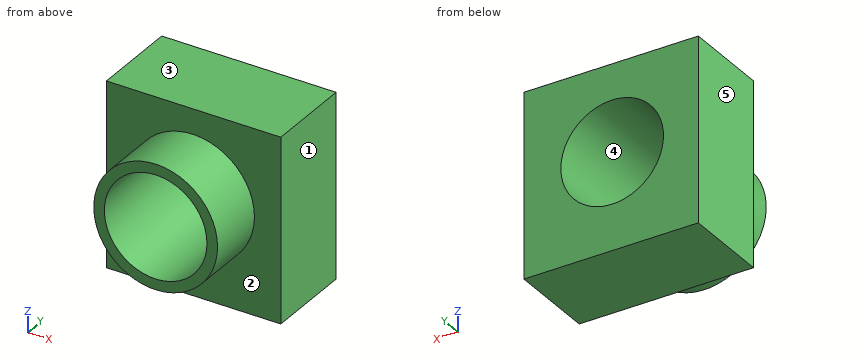
```python
from build123d import *

# Parameters (mm, degrees)
F0_W     = 75.738185
F0_H     = 79.894543
F1_DEPTH = 38.1
F2_R     = 26.877172
F3_DEPTH = 25.4
F4_R     = 22.28871
F5_DEPTH = 63.501


with BuildPart() as f1:
    # F0 (on Front) → F1 (new body)
    with BuildSketch(Plane.XZ):
        with Locations((0.46182, -2.193634)):
            Rectangle(F0_W, F0_H)
    extrude(amount=F1_DEPTH)

    # F2 (on face) → F3 (join)
    with BuildSketch(Plane.XZ.offset(38.1)):
        Circle(F2_R)
    extrude(amount=F3_DEPTH)

    # F4 (on face) → F5 (cut, through all)
    with BuildSketch(Plane.XZ.offset(63.5)):
        Circle(F4_R)
    extrude(amount=-F5_DEPTH, mode=Mode.SUBTRACT)


solid = f1.part
```
The listing builds one solid part. Answer for the finished solid, in the listing's coordinates (mm). Face numbers are marked on the shaded views. A direction names the side the tool comes from. Coordinates: 2 decimals unless noted, no trailing zeros. Loops run counter-clockwise (first coordinate to the right, second up) from the corner with the lowest first, then second, coordinate; pieces in that order, holes last. Notation, with made-up numbers: M 22,41 L 64,41 A8 ccw 64,53 Z; hole C 54,-12 d2. An arc over 180 degrees is marked long. Answer as a JSON object with one key per item and string values. Group by question number.
Item 1: Section C-C (y = -30.5) is taken. Write down the section's boundary in (x, z).
Item 2: Determine the mould class of the marked faces 3, 4 and 5 for opening direction X: +X half, -X half, draft (parallel to the pull), parting line (faces both ways), or undercut.
Item 3: Consider L1, parallel to Z at x = 0, y = -27.5; L2, parallel to Z at x = 0, y = -47.5; L3, parallel to X at y = -8.5, z = 16. Determine where each line is inside the solid, lowest interval first.
Item 4: Section B-B (x = 0) is taken. Write down the section's boundary in (y, z), and give its area (3 significant figures).
Item 5: Section D-D (x = 24) is taken. Write down the section's boundary in (y, z).
Item 6: Section A-A (z = 0) is taken. Write down the section's boundary in (x, y), and give its area (3 significant figures).
Item 7: Each of these flat-tipped pins is pushed along its axis until it touches: P1, Ø12, axis at x = 15, z = -32, coming from the -Y side; P2, Ø22.5, axis at x = -18.5, z = -20.5, coming from the -Y side; P3, Ø1.5, axis at y = -46.5, z = -22.5, coming from the +X side; P4, Ø1, axis at x = -14.5, z = -14, coming from the +Y side. Where does it stop, or does it pass through?
Item 8: Which of the six approach directions +Z, -Z, +X, -X, +Y, -Y give full straight-line access (tool end or side, diameter ignored) to the marked faces 1 and 2?
Solved:
{
 "1": {"outline": "M -37.41,-42.14 L 38.33,-42.14 L 38.33,37.75 L -37.41,37.75 Z; hole C 0,0 d44.58"},
 "2": {"face 3": "draft", "face 4": "undercut", "face 5": "-X half"},
 "3": {"L1": "z = -42.14 to -22.29, 22.29 to 37.75", "L2": "z = -26.88 to -22.29, 22.29 to 26.88", "L3": "x = -37.41 to -15.52, 15.52 to 38.33"},
 "4": {"outline": "M -63.5,-26.88 L -38.1,-26.88 L -38.1,-42.14 L 0,-42.14 L 0,-22.29 L -63.5,-22.29 Z; M -63.5,22.29 L 0,22.29 L 0,37.75 L -38.1,37.75 L -38.1,26.88 L -63.5,26.88 Z", "area": "1,580 mm2"},
 "5": {"outline": "M -63.5,-12.1 L -38.1,-12.1 L -38.1,-42.14 L 0,-42.14 L 0,37.75 L -38.1,37.75 L -38.1,12.1 L -63.5,12.1 Z"},
 "6": {"outline": "M -37.41,-38.1 L -26.88,-38.1 L -26.88,-63.5 L -22.29,-63.5 L -22.29,0 L -37.41,0 Z; M 22.29,-63.5 L 26.88,-63.5 L 26.88,-38.1 L 38.33,-38.1 L 38.33,0 L 22.29,0 Z", "area": "1,420 mm2"},
 "7": {"P1": "stops at y = -38.1", "P2": "stops at y = -63.5", "P3": "stops at x = 15.79", "P4": "passes through"},
 "8": {"face 1": "+Z, -Z, +X, +Y, -Y", "face 2": "-Y"}
}
